The model under review builds one solid part; all positions refer to its coordinate system, in mm. Face numbers are marked on the shaded views. A direction names the side the tool comes from. Give positions to 0.01 mm unless a question says otherwise; leave off trailing zeros. Write each loop counter-clockwise with the first axis right and the second up, starting at its lowest first coordinate (ties: lowest second). Pieces come first, ordered by that corner, then holes. Notation, with made-up numbers: (-13, 17) - (2, 17) arc R19 ccw to (2, 42) - close; hole circle Ø3 at (77, 74). An arc over 180 degrees is marked (long way). Write item = value, one per line.
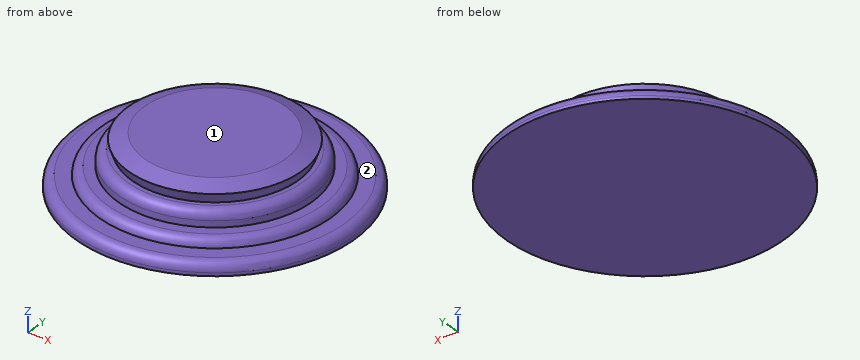
```python
from build123d import *

# Parameters (mm, degrees)
F0_R      = 77.7501635543
F0_R_2    = 64.6980648952
F1_DEPTH  = 6.858
F0_R_3    = 54.0479242204
F2_DEPTH  = 11.43
F0_R_4    = 39.0523448649
F3_DEPTH  = 20.066
F5_DEPTH  = 25.654
F5_TAPER  = -20
F5_FACE_R = 48.3896372547
F6_DEPTH  = 3.302
F6_TAPER  = 70


# Not quite as in the source:
# - a fillet or chamfer that OpenCascade refuses, or shapes differently, is made with other operations: its cross-section is extruded or revolved along the edge and cut away or added


with BuildPart() as f1:
    # F0 (on Top) → F1 (new body)
    with BuildSketch(Plane.XY):
        Circle(F0_R)
        Circle(F0_R_2, mode=Mode.SUBTRACT)
    extrude(amount=F1_DEPTH)

    # F0 (on Top) → F2 (join)
    with BuildSketch(Plane.XY):
        Circle(F0_R_2)
        Circle(F0_R_3, mode=Mode.SUBTRACT)
    extrude(amount=F2_DEPTH)

    # F0 (on Top) → F3 (join)
    with BuildSketch(Plane.XY):
        Circle(F0_R_3)
        Circle(F0_R_4, mode=Mode.SUBTRACT)
    extrude(amount=F3_DEPTH)

    # F4: fillet of radius 5.08 on 3 edges, made by hand

    # F4_s1 → F4_t2 (revolve, cut)
    with BuildSketch(Plane.XZ):
        with BuildLine():
            ThreePointArc((48.9679242204, 20.066), (52.5600266688, 18.5781024484), (54.0479242204, 14.986))
            Line((54.0479242204, 14.986), (54.0479242204, 20.066))
            Line((54.0479242204, 20.066), (48.9679242204, 20.066))
        make_face()
    revolve(axis=Axis((0, 0, 20.066), (0, 0, 1)), mode=Mode.SUBTRACT)

    # F4_s3 → F4_t4 (revolve, cut)
    with BuildSketch(Plane.XZ):
        with BuildLine():
            ThreePointArc((64.6980648952, 6.858), (63.0512963124, 10.1174288314), (59.6435287147, 11.43))
            Line((59.6435287147, 11.43), (64.6980648952, 11.43))
            Line((64.6980648952, 11.43), (64.6980648952, 6.858))
        make_face()
    revolve(axis=Axis((0, 0, 11.43), (0, 0, 1)), mode=Mode.SUBTRACT)

    # F4_s5 → F4_t6 (revolve, cut)
    with BuildSketch(Plane.XZ):
        with BuildLine():
            ThreePointArc((77.7501635543, 1.778), (76.2622660027, 5.3701024484), (72.6701635543, 6.858))
            Line((72.6701635543, 6.858), (77.7501635543, 6.858))
            Line((77.7501635543, 6.858), (77.7501635543, 1.778))
        make_face()
    revolve(axis=Axis((0, 0, 6.858), (0, 0, 1)), mode=Mode.SUBTRACT)

    # F0 (on Top) → F5 (join)
    with BuildSketch(Plane.XY):
        Circle(F0_R_4)
    extrude(amount=F5_DEPTH, taper=F5_TAPER)

    # F5_face (on face) → F6 (join)
    with BuildSketch(Plane.XY.offset(25.654)):
        Circle(F5_FACE_R)
    extrude(amount=F6_DEPTH, taper=F6_TAPER)


solid = f1.part
```
1. Insertion check: P1, Ø1, axis at y = 2.5, z = 14.5, coming from the +X side; P2, Ø1.5, axis at y = -17.5, z = 8, coming from the +X side; P3, Ø1, axis at x = -38.5, y = -46, coming from the +Z side. Each pin has a flat end and moves straight along its axis. Give the tip position at first contact, or say it passes through.
Findings below:
P1 = 54.01
P2 = 62.33
P3 = 11.43
2. Machinability: for the marked faces 1 and 2, which of the approach directions +Z, -Z, +X, -X, +Y, -Y give a long, thin tool a straight path to every point of the face, cutting with its end or side? Answer none if there is none.
Findings below:
face_1 = +Z, +X, -X, +Y, -Y
face_2 = +Z
3. Take a section at C-C on z = 23.75. Give the boundary of the cut face in (x, y), and give its area (3 significant figures).
Findings below:
outline = circle Ø95.39 at (0, 0)
area = 7,150 mm²
4. Take a section at A-A on x = 0. Give the boundary of the cut face in (y, z).
Findings below:
outline = (-77.75, 0) - (77.75, 0) - (77.75, 1.78) arc R5.08 ccw to (72.67, 6.86) - (64.7, 6.86) arc R5.08 ccw to (59.64, 11.43) - (54.05, 11.43) - (54.05, 14.99) arc R5.08 ccw to (48.97, 20.07) - (46.36, 20.07) - (48.39, 25.65) - (39.32, 28.96) - (-39.32, 28.96) - (-48.39, 25.65) - (-46.36, 20.07) - (-48.97, 20.07) arc R5.08 ccw to (-54.05, 14.99) - (-54.05, 11.43) - (-59.64, 11.43) arc R5.08 ccw to (-64.7, 6.86) - (-72.67, 6.86) arc R5.08 ccw to (-77.75, 1.78) - close
5. For line 1 (Z direction, x = -69.5, y = -18); line 2 (X direction, y = -41, z = 25.5); line 3 (Z direction, x = -38, y = -12), list the stretches that pass through material, from the lowest coordinate up. Write a range as from..to.
Findings below:
line_1 = 0..6.86
line_2 = -25.6..25.6
line_3 = 0..28.76
6. Take a section at B-B on z = 9. Give the boundary of the cut face in (x, y), and give its area (3 significant figures).
Findings below:
outline = circle Ø127.96 at (0, 0)
area = 12,900 mm²
